Autodesk Inventor part; units mm, degrees
ref_plane "YZ Plane" through (0, 0, 0) normal (1, 0, 0) x (0, 1, 0)
ref_plane "XZ Plane" through (0, 0, 0) normal (0, 1, 0) x (-1, 0, 0)
ref_plane "XY Plane" through (0, 0, 0) normal (0, 0, 1) x (1, 0, 0)
sketch "Sketch1" plane through (0, 0, 0) normal (0, 1, 0) x (-1, 0, 0)
  line L0 (0, 0) -> (0, -15) construction
  line L1 (-3.5, 0) -> (-3.5, -15)
  line L2 (3.5, -15) -> (3.5, 0)
  arc A0 (3.5, 0) -> (-3.5, 0) centre (0, 0) ccw
  arc A1 (-3.5, -15) -> (3.5, -15) centre (0, -15) ccw
  circle A2 centre (0, 0) radius 1.7
  point P0 (0, -7.5)
  dimension "d0" = 7
  dimension "d1" = 15
  dimension "d2" = 3.4
extrude "Extrusion1" add sketch "Sketch1" along normal blind 5
sketch "Sketch2" plane through (0, 5, 0) normal (0, 1, 0) x (1, 0, 0)
  circle A0 centre (0, 0) radius 2.625
  dimension "d5" = 5.25
extrude "Extrusion2" cut sketch "Sketch2" against normal blind 3
fillet "Fillet1" radius 0.5 8 edges at (0, 0, -18.5) (-3.5, 0, -7.5) (0, 0, 3.5) (3.5, 0, -7.5) (0, 5, -18.5) (-3.5, 5, -7.5) (0, 5, 3.5) (3.5, 5, -7.5)
properties part number "v2batterylock"
For this review, take the finished solid that the model builds, in its own axes (mm). A direction names the side the tool comes from. Give positions to 0.01 mm unless a question says otherwise; leave off trailing zeros. Order: outer loops, then holes, each group sorted by start corner. A loop starts at its lowest first (then second) coordinate and runs counter-clockwise, first axis right, second up. Notation, with made-up numbers: (42.5, 10) -> (101.5, 10) arc R27 ccw to (101.5, 43) -> close; hole circle Ø2 at (76.5, 73.5). An arc over 180 degrees is marked (long way). Write item = value, one per line.
1) For faces 1 (the face through (0, 5, -10)), 2 (the face through (2.5, 3.5, -0.8)), list the 3-axis set-ups (+Z, -Z, +X, -X, +Y, -Y) from which the entire face can be reached by the end or side of a thin tool; tool diameter is ignored.
Findings:
face_1 = +Z, -Z, +X, -X, +Y
face_2 = +Y
2) Draft analysis for pull direction Z (two halves, no side actions). For faces 3 (the face through (0, 2, 2)), 4 (the face through (-0.1, 2.5, -18.5)), 5 (the face through (3.5, 2, -7)), 6 (the face through (0.37, 0.99, 1.66)), state which applies: pulls with the +Z half, pulls with the -Z half, needs draft (parallel to the pull), parting line crosses it, or undercut.
Findings:
face_3 = undercut
face_4 = pulls with the -Z half
face_5 = needs draft
face_6 = undercut
3) To check wall thickness, follow L1, parallel to Z at x = 0, y = 0.5; L2, parallel to Z at x = 0, y = 2.85 (3 decimals); L3, parallel to X at y = 3.95, z = 0 (3 decimals). State the ranges of each line that lie inside material, in increasing order. Write a range as from..to.
Findings:
L1 = -18.5..-1.7, 1.7..3.5
L2 = -18.5..-2.625, 2.625..3.5
L3 = -3.5..-2.625, 2.625..3.5
4) Insertion check: pin 1 (2.5 mm diameter, centred on x = 0, z = 0, fed in from +Y); pin 2 (2.5 mm diameter, centred on x = -0.5, z = -0.5, fed in from +Y). Each pin has a flat end and moves straight along its axis. Give the tip position at first contact, or say it passes through.
Findings:
pin_1 = through
pin_2 = 2
5) We need section C-C, the plane y = 2.25. Give the boundary of the cut face in (x, z) (3 decimals).
Findings:
outline = (-3.5, -15) arc R3.5 ccw to (3.5, -15) -> (3.5, 0) arc R3.5 ccw to (-3.5, 0) -> close; hole circle Ø5.25 at (0, 0)
6) We need section B-B, the plane x = 0. Give the boundary of the cut face in (y, z) (3 decimals), and give its area (3 significant figures).
Findings:
outline = (0, -18) arc R0.5 ccw to (0.5, -18.5) -> (4.5, -18.5) arc R0.5 ccw to (5, -18) -> (5, -2.625) -> (2, -2.625) -> (2, -1.7) -> (0, -1.7) -> close; (0, 1.7) -> (2, 1.7) -> (2, 2.625) -> (5, 2.625) -> (5, 3) arc R0.5 ccw to (4.5, 3.5) -> (0.5, 3.5) arc R0.5 ccw to (0, 3) -> close
area = 87.2 mm^2
7) We need section A-A, the plane y = 0.7. Give the boundary of the cut face in (x, z).
Findings:
outline = (-3.5, -15) arc R3.5 ccw to (3.5, -15) -> (3.5, 0) arc R3.5 ccw to (-3.5, 0) -> close; hole circle Ø3.4 at (0, 0)
